Build history of the part. All positions in model axes, mm. A direction names the side the tool comes from. Coordinates: 2 decimals unless noted, no trailing zeros. Write each loop counter-clockwise with the first axis right and the second up, starting at its lowest first coordinate (ties: lowest second). Pieces come first, ordered by that corner, then holes. Notation, with made-up numbers: (-6, 51.25) -> (6, 51.25) arc R33 ccw to (6, 90.25) -> close; hole circle Ø3 at (41, 57). An arc over 180 degrees is marked (long way). Write each question's results on one line, items separated by ' | '. Start each with the question number.
Q1. Saw through at D-D on y = 12. Give the cut face in (x, z), and give its area (3 significant figures).
Q2. Saw through at A-A on x = 0. Give the cut face in (y, z).
Q3. Two-plate mould, pull along Z, no slides. Class faces 1 (the face through (6.466, 9.86, -2.681)), 2 (the face through (0, 40, -6)), 3 (the face through (-14.985, 19.734, 0.66)): released by +Z, released by -Z, zero draft, split by the parting line, or undercut.
Q4. Saw through at C-C on y = 30. Give the cut face in (x, z).
Q5. Drop flat-ended pins along their axis: pin 1 Ø7 at (x, z) = (-1.5, -1.5) entering from -Y; pin 2 Ø8 at (y, z) = (16.5, 10) entering from +X; pin 3 Ø5 at (y, z) = (7.5, -5) entering from -X. Give the stop position or say it passes through.
Q6. Saw through at B-B on z = 0. Give the cut face in (x, y).
Q7. Drill centre lines: line 1 (Z direction, x = 0, y = 28); line 2 (Y direction, x = 0, z = -6.5); line 3 (X direction, y = 3, z = 4.5). Where is each one in solid material? Low to high.
Q8. Tool access for faces 4 (the face through (-6.4, 0, 3.3)), 5 (the face through (-2, 20, 5)): list every direction of +Z, -Z, +X, -X, +Y, -Y with a clear straight run to the whole face (end or side of a thin tool).
from build123d import *

# Parameters (mm, degrees)
F6_R     = 15
F0_DEPTH = 40
F1_R     = 1
F2_R     = 7
F3_DEPTH = 20
F4_R     = 5
F5_DEPTH = 20


with BuildPart() as f0:
    # F6 (on Front) → F0 (new body)
    with BuildSketch(Plane.XZ):
        Circle(F6_R)
    extrude(amount=-F0_DEPTH)

    # F1
    f1_edges = [f0.edges().sort_by_distance(p)[0] for p in [
        (-15, 0, 0),
        (-15, 40, 0),
    ]]
    fillet(f1_edges, radius=F1_R)

    # F2 (on face) → F3 (cut)
    with BuildSketch(Plane.XZ):
        Circle(F2_R)
    extrude(amount=-F3_DEPTH, mode=Mode.SUBTRACT)

    # F4 (on face) → F5 (cut)
    with BuildSketch(Plane(origin=(0, 40, 0), x_dir=(-1, 0, 0), z_dir=(0, 1, 0))):
        Circle(F4_R)
    extrude(amount=-F5_DEPTH, mode=Mode.SUBTRACT)


solid = f0.part
Returned:
1) outline: circle Ø30 at (0, 0); hole circle Ø14 at (0, 0) | area: 553 mm2
2) outline: (0, -14) arc R1 ccw to (1, -15) -> (39, -15) arc R1 ccw to (40, -14) -> (40, -5) -> (20, -5) -> (20, -7) -> (0, -7) -> close; (0, 7) -> (20, 7) -> (20, 5) -> (40, 5) -> (40, 14) arc R1 ccw to (39, 15) -> (1, 15) arc R1 ccw to (0, 14) -> close
3) face 1: undercut | face 2: zero draft | face 3: split by the parting line
4) outline: circle Ø30 at (0, 0); hole circle Ø10 at (0, 0)
5) pin 1: stops at y = 20 | pin 2: stops at x = 13.75 | pin 3: stops at x = -14.79
6) outline: (-15, 1) arc R1 ccw to (-14, 0) -> (-7, 0) -> (-7, 20) -> (-5, 20) -> (-5, 40) -> (-14, 40) arc R1 ccw to (-15, 39) -> close; (5, 20) -> (7, 20) -> (7, 0) -> (14, 0) arc R1 ccw to (15, 1) -> (15, 39) arc R1 ccw to (14, 40) -> (5, 40) -> close
7) line 1: z = -15 to -5, 5 to 15 | line 2: y = 20 to 40 | line 3: x = -14.31 to -5.36, 5.36 to 14.31
8) face 4: +Z, -Z, +X, -X, -Y | face 5: -Y
